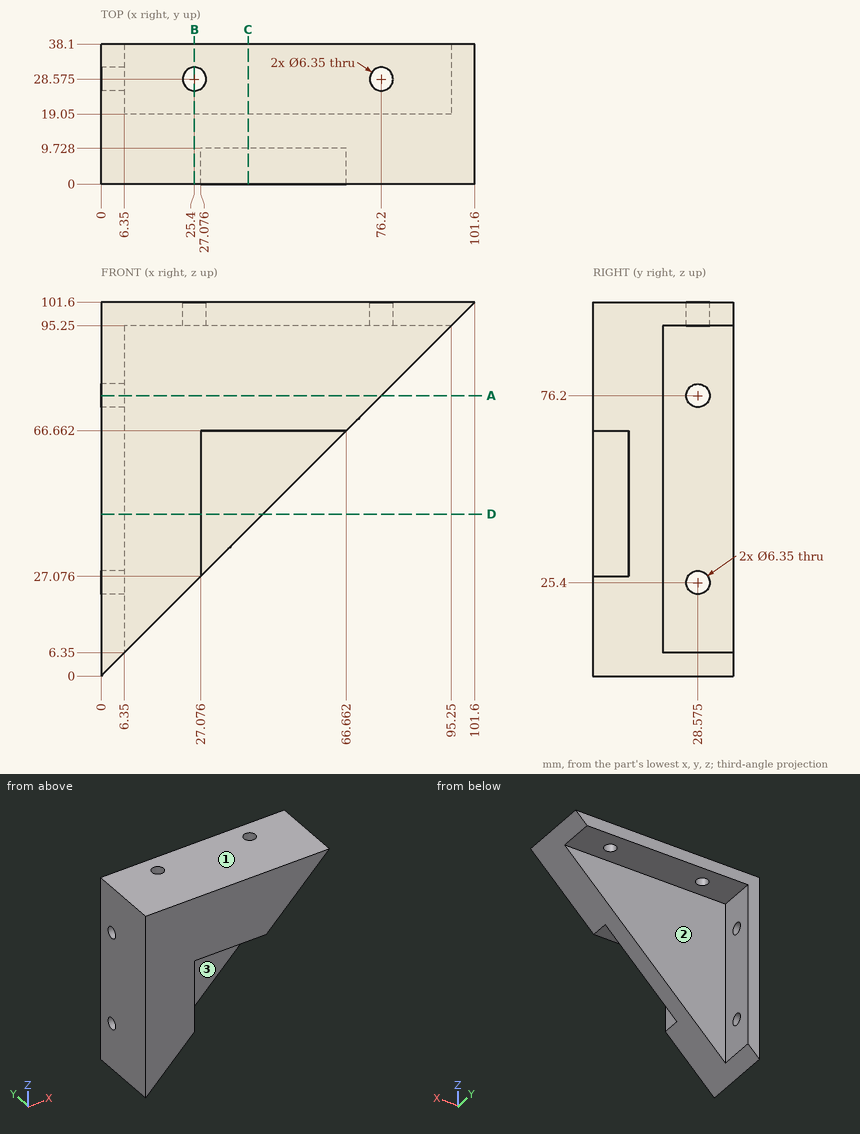
The drawing under review shows one solid part. Ordinate dimensions are in mm from its lowest x, y, z. A direction names the side the tool comes from. Coordinates: 2 decimals unless noted, no trailing zeros. Order: outer loops, then holes, each group sorted by start corner. A loop starts at its lowest first (then second) coordinate and runs counter-clockwise, first axis right, second up. Notation, with made-up numbers: M -6,-36.75 L 19,-36.75 A22 cw 19,-17.75 Z; hole C -19,-15.5 d4. An arc over 180 degrees is marked long. One line per question, with ' | ' between items.
(1) Insertion check: pin 1 (10 mm diameter, centred on y = 11.5, z = 42.5, fed in from +X); pin 2 (5 mm diameter, centred on y = 5, z = 42, fed in from +X); pin 3 (5 mm diameter, centred on y = 17, z = 33.5, fed in from +X). Each pin has a flat end and moves straight along its axis. Give the tip position at first contact, or say it passes through.
Geometry results:
pin 1: stops at x = 47.5 | pin 2: stops at x = 27.08 | pin 3: stops at x = 36
(2) Add section C-C, the plane x = 40. Write out the cut boundary in (y, z).
Geometry results:
outline: M 0,66.66 L 9.73,66.66 L 9.73,40 L 19.05,40 L 19.05,95.25 L 38.1,95.25 L 38.1,101.6 L 0,101.6 Z
(3) Add section B-B, the plane x = 25.4. Write out the cut boundary in (y, z), then the cut area to 3 significant figures.
Geometry results:
outline: M 0,25.4 L 19.05,25.4 L 19.05,95.25 L 25.4,95.25 L 25.4,101.6 L 0,101.6 Z; M 31.75,95.25 L 38.1,95.25 L 38.1,101.6 L 31.75,101.6 Z | area: 1,530 mm²
(4) Add section D-D, the plane z = 44. Write out the cut boundary in (x, y).
Geometry results:
outline: M 0,0 L 27.08,0 L 27.08,9.73 L 44,9.73 L 44,19.05 L 6.35,19.05 L 6.35,38.1 L 0,38.1 Z
(5) Add section A-A, the plane z = 76.2. Write out the cut boundary in (x, y), then the cut area to 3 significant figures.
Geometry results:
outline: M 0,0 L 76.2,0 L 76.2,19.05 L 6.35,19.05 L 6.35,25.4 L 0,25.4 Z; M 0,31.75 L 6.35,31.75 L 6.35,38.1 L 0,38.1 Z | area: 1,530 mm²
(6) Machinability: for the marked faces 1, 2 and 3, which of the approach directions +Z, -Z, +X, -X, +Y, -Y give a long, thin tool a straight path to every point of the face, cutting with its end or side? Answer none if there is none.
Geometry results:
face 1: +Z, +X, -X, +Y, -Y | face 2: -Z, +X, +Y | face 3: -Z, +X, -Y
(7) For probe 1 along Y at (x, z) = (4, 76.2); probe 2 along X at (y, z) = (28, 71); probe 3 along Z at (x, y) = (45, 7.5), list the stretches that pass through material, from the lowest coordinate up. Write a range as from..to.
Geometry results:
probe 1: y = 0..25.4, 31.75..38.1 | probe 2: x = 0..6.35 | probe 3: z = 66.66..101.6
